Verification items for the finished model (mm, model axes). Face numbers are marked on the shaded views. A direction names the side the tool comes from. Give positions to 0.01 mm unless a question says otherwise; leave off trailing zeros. Loops run counter-clockwise (first coordinate to the right, second up) from the corner with the lowest first, then second, coordinate; pieces in that order, holes last. Notation, with made-up numbers: (-19, 4.5) -> (10, 4.5) arc R16 ccw to (10, 28.5) -> close; hole circle Ø2 at (2, -12.5). An arc over 180 degrees is marked (long way). Answer in a Markdown table with one row per item. Add a question column.
Q1. Set-up check for the marked faces 4, 5, 6, 7 and 8: record each of +Z, -Z, +X, -X, +Y, -Y from which the full face is reachable in a straight line by a thin tool's end or side.
Q2. Release check for a two-part mould opening along Y. For the marked faces 1, 2 and 3 record: pulls with the +Y half, pulls with the -Y half, needs draft (parallel to the pull), parting line crosses it, or undercut.
Q3. Gauge pin test, flat ends, axial feed: P1, Ø5, axis at y = 42, z = 4.5, coming from the -X side; P2, Ø2, axis at x = 40.5, z = 5, coming from the -Y side; P3, Ø2, axis at x = 13.5, z = 5.5, coming from the -Y side. Record the tip position at first contact, or that the pin passes through.
Q4. Material ranges on probe 1 along X at (y, z) = (42, 4.5); probe 2 along Y at (x, z) = (0, 7.5); probe 3 along Y at (x, z) = (59, 3.5), recorded low to high.
Q5. Section check A-A on y = -33. Enter the section's corners in (x, z), and give its area (3 significant figures).
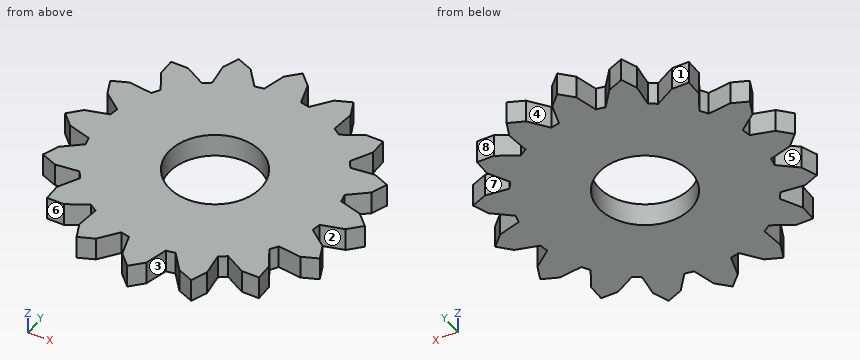
```python
from build123d import *

# Parameters (mm, degrees)
BOSS_EXTRUDE2_DEPTH = 10
SKETCH2_R           = 20
CUT_EXTRUDE1_DEPTH  = 10


with BuildPart() as part:
    # Sketch1 → Boss-Extrude2 (new body)
    with BuildSketch(Plane.XY):
        with BuildLine():
            Line((17.811997012, 56.458001404), (11.62649389, 48.629462673))
            ThreePointArc((11.62649389, 48.629462673), (9.754516101, 49.03926402), (7.86820995, 49.377031828))
            Line((7.86820995, 49.377031828), (5.14940229, 58.976748098))
            Line((5.14940229, 58.976748098), (0, 64.126150387))
            Line((0, 64.126150387), (-5.14940229, 58.976748098))
            Line((-5.14940229, 58.976748098), (-7.86820995, 49.377031828))
            ThreePointArc((-7.86820995, 49.377031828), (-9.754516101, 49.03926402), (-11.62649389, 48.629462673))
            Line((-11.62649389, 48.629462673), (-17.811997012, 56.458001404))
            Line((-17.811997012, 56.458001404), (-24.540015335, 59.244837841))
            Line((-24.540015335, 59.244837841), (-27.326851772, 52.516819519))
            Line((-27.326851772, 52.516819519), (-26.16505015, 42.607395492))
            ThreePointArc((-26.16505015, 42.607395492), (-27.778511651, 41.573480615), (-29.351169429, 40.478498652))
            Line((-29.351169429, 40.478498652), (-38.061681234, 45.34403579))
            Line((-38.061681234, 45.34403579), (-45.34403579, 45.34403579))
            Line((-45.34403579, 45.34403579), (-45.34403579, 38.061681234))
            Line((-45.34403579, 38.061681234), (-40.478498652, 29.351169429))
            ThreePointArc((-40.478498652, 29.351169429), (-41.573480615, 27.778511651), (-42.607395492, 26.16505015))
            Line((-42.607395492, 26.16505015), (-52.516819519, 27.326851772))
            Line((-52.516819519, 27.326851772), (-59.244837841, 24.540015335))
            Line((-59.244837841, 24.540015335), (-56.458001404, 17.811997012))
            Line((-56.458001404, 17.811997012), (-48.629462673, 11.62649389))
            ThreePointArc((-48.629462673, 11.62649389), (-49.03926402, 9.754516101), (-49.377031828, 7.86820995))
            Line((-49.377031828, 7.86820995), (-58.976748098, 5.14940229))
            Line((-58.976748098, 5.14940229), (-64.126150387, 0))
            Line((-64.126150387, 0), (-58.976748098, -5.14940229))
            Line((-58.976748098, -5.14940229), (-49.377031828, -7.86820995))
            ThreePointArc((-49.377031828, -7.86820995), (-49.03926402, -9.754516101), (-48.629462673, -11.62649389))
            Line((-48.629462673, -11.62649389), (-56.458001404, -17.811997012))
            Line((-56.458001404, -17.811997012), (-59.244837841, -24.540015335))
            Line((-59.244837841, -24.540015335), (-52.516819519, -27.326851772))
            Line((-52.516819519, -27.326851772), (-42.607395492, -26.16505015))
            ThreePointArc((-42.607395492, -26.16505015), (-41.573480615, -27.778511651), (-40.478498652, -29.351169429))
            Line((-40.478498652, -29.351169429), (-45.34403579, -38.061681234))
            Line((-45.34403579, -38.061681234), (-45.34403579, -45.34403579))
            Line((-45.34403579, -45.34403579), (-38.061681234, -45.34403579))
            Line((-38.061681234, -45.34403579), (-29.351169429, -40.478498652))
            ThreePointArc((-29.351169429, -40.478498652), (-27.778511651, -41.573480615), (-26.16505015, -42.607395492))
            Line((-26.16505015, -42.607395492), (-27.326851772, -52.516819519))
            Line((-27.326851772, -52.516819519), (-24.540015335, -59.244837841))
            Line((-24.540015335, -59.244837841), (-17.811997012, -56.458001404))
            Line((-17.811997012, -56.458001404), (-11.62649389, -48.629462673))
            ThreePointArc((-11.62649389, -48.629462673), (-9.754516101, -49.03926402), (-7.86820995, -49.377031828))
            Line((-7.86820995, -49.377031828), (-5.14940229, -58.976748098))
            Line((-5.14940229, -58.976748098), (0, -64.126150387))
            Line((0, -64.126150387), (5.14940229, -58.976748098))
            Line((5.14940229, -58.976748098), (7.86820995, -49.377031828))
            ThreePointArc((7.86820995, -49.377031828), (9.754516101, -49.03926402), (11.62649389, -48.629462673))
            Line((11.62649389, -48.629462673), (17.811997012, -56.458001404))
            Line((17.811997012, -56.458001404), (24.540015335, -59.244837841))
            Line((24.540015335, -59.244837841), (27.326851772, -52.516819519))
            Line((27.326851772, -52.516819519), (26.16505015, -42.607395492))
            ThreePointArc((26.16505015, -42.607395492), (27.778511651, -41.573480615), (29.351169429, -40.478498652))
            Line((29.351169429, -40.478498652), (38.061681234, -45.34403579))
            Line((38.061681234, -45.34403579), (45.34403579, -45.34403579))
            Line((45.34403579, -45.34403579), (45.34403579, -38.061681234))
            Line((45.34403579, -38.061681234), (40.478498652, -29.351169429))
            ThreePointArc((40.478498652, -29.351169429), (41.573480615, -27.778511651), (42.607395492, -26.16505015))
            Line((42.607395492, -26.16505015), (52.516819519, -27.326851772))
            Line((52.516819519, -27.326851772), (59.244837841, -24.540015335))
            Line((59.244837841, -24.540015335), (56.458001404, -17.811997012))
            Line((56.458001404, -17.811997012), (48.629462673, -11.62649389))
            ThreePointArc((48.629462673, -11.62649389), (49.03926402, -9.754516101), (49.377031828, -7.86820995))
            Line((49.377031828, -7.86820995), (58.976748098, -5.14940229))
            Line((58.976748098, -5.14940229), (64.126150387, 0))
            Line((64.126150387, 0), (58.976748098, 5.14940229))
            Line((58.976748098, 5.14940229), (49.377031828, 7.86820995))
            ThreePointArc((49.377031828, 7.86820995), (49.03926402, 9.754516101), (48.629462673, 11.62649389))
            Line((48.629462673, 11.62649389), (56.458001404, 17.811997012))
            Line((56.458001404, 17.811997012), (59.244837841, 24.540015335))
            Line((59.244837841, 24.540015335), (52.516819519, 27.326851772))
            Line((52.516819519, 27.326851772), (42.607395492, 26.16505015))
            ThreePointArc((42.607395492, 26.16505015), (41.573480615, 27.778511651), (40.478498652, 29.351169429))
            Line((40.478498652, 29.351169429), (45.34403579, 38.061681234))
            Line((45.34403579, 38.061681234), (45.34403579, 45.34403579))
            Line((45.34403579, 45.34403579), (38.061681234, 45.34403579))
            Line((38.061681234, 45.34403579), (29.351169429, 40.478498652))
            ThreePointArc((29.351169429, 40.478498652), (27.778511651, 41.573480615), (26.16505015, 42.607395492))
            Line((26.16505015, 42.607395492), (27.326851772, 52.516819519))
            Line((27.326851772, 52.516819519), (24.540015335, 59.244837841))
            Line((24.540015335, 59.244837841), (17.811997012, 56.458001404))
        make_face()
    extrude(amount=BOSS_EXTRUDE2_DEPTH)

    # Sketch2 → Cut-Extrude1 (cut)
    with BuildSketch(Plane(origin=(0, 0, 0), x_dir=(-1, 0, 0), z_dir=(0, 0, -1))):
        Circle(SKETCH2_R)
    extrude(amount=-CUT_EXTRUDE1_DEPTH, mode=Mode.SUBTRACT)


solid = part.part
```
Taken from the geometry:
| question | item | result |
|---|---|---|
| 1 | face 4 | +Z, -Z, +Y |
| 1 | face 5 | +Z, -Z, -X |
| 1 | face 6 | +Z, -Z, -X, -Y |
| 1 | face 7 | +Z, -Z |
| 1 | face 8 | +Z, -Z, +X, +Y |
| 2 | face 1 | pulls with the +Y half |
| 2 | face 2 | undercut |
| 2 | face 3 | pulls with the -Y half |
| 3 | P1 | stops at x = -45.34 |
| 3 | P2 | stops at y = -45.34 |
| 3 | P3 | stops at y = -52.27 |
| 4 | probe 1 | x = -45.34 to -32.08, -27.13 to 27.13, 32.08 to 45.34 |
| 4 | probe 2 | y = -64.13 to -20, 20 to 64.13 |
| 4 | probe 3 | y = -24.64 to -23.95, -5.13 to 5.13, 23.95 to 24.64 |
| 5 | outline | (-42.52, 0) -> (42.52, 0) -> (42.52, 10) -> (-42.52, 10) -> close |
| 5 | area | 850 mm² |
